from build123d import *

# Parameters (mm, degrees)
F0_W     = 233.420394361
F0_H     = 166.5441393852
F1_DEPTH = 1.27
F2_DEPTH = 0.254
F3_DEPTH = 25.4
F4_W     = 69.0996274352
F4_H     = 38.4067334235
F5_DEPTH = 2.54


with BuildPart() as f1:
    # F0 (on Front) → F1 (new body)
    with BuildSketch(Plane.XZ):
        with Locations((1.6535334289, -5.4845437407)):
            Rectangle(F0_W, F0_H)
    extrude(amount=F1_DEPTH)

    # F2 (add): a face of the model
    f2_faces = [f1.faces().sort_by_distance(p)[0] for p in [
        (1.6535334289, -1.27, -5.4845437407),
    ]]
    extrude(f2_faces, amount=F2_DEPTH)

    # F3 (add): a face of the model
    f3_faces = [f1.faces().sort_by_distance(p)[0] for p in [
        (1.6535334289, -1.524, -5.4845437407),
    ]]
    extrude(f3_faces, amount=F3_DEPTH)

    # F4 (on Top) → F5 (join)
    with BuildSketch(Plane.XY):
        with Locations((-6.8230740726, 19.2033667117)):
            Rectangle(F4_W, F4_H)
    extrude(amount=F5_DEPTH)


solid = f1.part
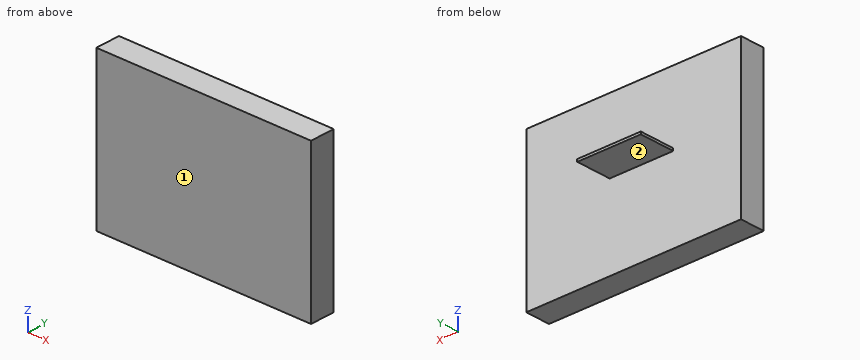
Verification items for the finished model (mm, model axes). Face numbers are marked on the shaded views. A direction names the side the tool comes from. Coordinates: 2 decimals unless noted, no trailing zeros. Write each loop counter-clockwise with the first axis right and the second up, starting at its lowest first coordinate (ties: lowest second). Pieces come first, ordered by that corner, then holes. Notation, with made-up numbers: (19.5, -39.75) - (69.5, -39.75) arc R23 cw to (69.5, -10.75) - close; hole circle Ø10 at (72, -26). An arc over 180 degrees is marked (long way). Answer as a JSON object with one key per item and string values.
(1) Gauge pin test, flat ends, axial feed: pin 1 Ø1.3 at (y, z) = (11, 1.5) entering from +X; pin 2 Ø0.8 at (y, z) = (19, 1.5) entering from -X; pin 3 Ø1.5 at (x, y) = (-8, 31) entering from -Z. Record the tip position at first contact, or that the pin passes through.
Report:
{"pin 1": "x = 27.73", "pin 2": "x = -41.37", "pin 3": "z = 0"}
(2) Cross-section at A-A on x = -17.5. Record the cut outline in (y, z), plus the area to 3 significant figures.
Report:
{"outline": "(-26.92, -88.76) - (0, -88.76) - (0, 0) - (38.41, 0) - (38.41, 2.54) - (0, 2.54) - (0, 77.79) - (-26.92, 77.79) - close", "area": "4,580 mm^2"}
(3) Cross-section at B-B on y = 24.5. Record the cut outline in (x, z), plus the area to 3 significant figures.
Report:
{"outline": "(-41.37, 0) - (27.73, 0) - (27.73, 2.54) - (-41.37, 2.54) - close", "area": "176 mm^2"}
(4) Cross-section at C-C on z = 16.5. Record the cut outline in (x, y), plus the area to 3 significant figures.
Report:
{"outline": "(-115.06, -26.92) - (118.36, -26.92) - (118.36, 0) - (-115.06, 0) - close", "area": "6,280 mm^2"}
(5) Tool access check on the marked faces 1 and 2. Record the directions out of +Z, -Z, +X, -X, +Y, -Y that give a thin tool (end or side, any length) a straight path to the whole face; none if there is none.
Report:
{"face 1": "+Z, -Z, +X, -X, -Y", "face 2": "-Z, +X, -X, +Y"}
(6) Thickness scan on line 1 along Y through (x, z) = (-68.5, 22.5); line 2 along Z through (x, y) = (26, 11.5). Record the ranges inside material, lowest first.
Report:
{"line 1": "-26.92 to 0", "line 2": "0 to 2.54"}
